from build123d import *

# Parameters (mm, degrees)
EXTRUDE_1_DEPTH             = 3
SKETCH_2_R                  = 1.5
CUT_EXTRUDE_1_DEPTH         = 158.429349233
FILLET_1_R                  = 10
FILLET_2_R                  = 2
HOLE_WIZARD_M3_1_AT_2_COUNT = 2
HOLE_WIZARD_M3_1_AT_2_PITCH = 20


with BuildPart() as part:
    # 草图1 → 凸台-拉伸1 (new body)
    with BuildSketch(Plane.XY):
        Polygon((0, 0), (130, 0), (65, 88.741196746), align=None)
    extrude(amount=EXTRUDE_1_DEPTH)

    # 草图2 → 切除-拉伸1 (cut, through all)
    with BuildSketch(Plane.XY.offset(3)):
        with Locations((42.987595979, 36.688780191)):
            Circle(SKETCH_2_R)
        with Locations(Location((31.169414161, 20.554017147, 0), (0, 0, 180))):
            Circle(SKETCH_2_R)
    extrude(amount=-CUT_EXTRUDE_1_DEPTH, mode=Mode.SUBTRACT)

    # 圆角1
    fillet_1_edges = [part.edges().sort_by_distance(p)[0] for p in [
        (0, 0, 1.5),
    ]]
    fillet(fillet_1_edges, radius=FILLET_1_R)

    # 圆角2
    fillet_2_edges = [part.edges().sort_by_distance(p)[0] for p in [
        (65, 88.741196746, 1.5),
        (130, 0, 1.5),
    ]]
    fillet(fillet_2_edges, radius=FILLET_2_R)

    # 草图6 → M3 六角凹锥坑螺钉的锥形沉头孔1 (revolve, cut)
    with BuildSketch(Plane(origin=(42.987595979, 36.688780191, 3), x_dir=(0, -1, 0), z_dir=(1, 0, 0))):
        Polygon((0, 0), (0, 3), (1.7, 3), (1.7, 1.66), (3.36, 0), align=None)
    hole_wizard_m3_1 = revolve(axis=Axis((42.987595979, 36.688780191, 9.35), (0, 0, -1)), mode=Mode.SUBTRACT)

    # M3 六角凹锥坑螺钉的锥形沉头孔1 at 2: M3 六角凹锥坑螺钉的锥形沉头孔1 ×2
    with Locations(*[Vector(-0.5909090909090912, -0.8067381522408567, 0) * (i * HOLE_WIZARD_M3_1_AT_2_PITCH) for i in range(1, HOLE_WIZARD_M3_1_AT_2_COUNT)]):
        add(hole_wizard_m3_1, mode=Mode.SUBTRACT)


solid = part.part
Geometry: final body of the model. Coordinates: model frame, mm. Give positions to 0.01 mm unless a question says otherwise; leave off trailing zeros. Write each loop counter-clockwise with the first axis right and the second up, starting at its lowest first coordinate (ties: lowest second). Pieces come first, ordered by that corner, then holes.
(1) Cut plane A-A, the plane z = 2.5. Return loops of the section in (x, y), then the cut area to 3 significant figures.
(2) Cut plane C-C, the plane x = 118. Return loops of the section in (y, z), then the cut area to 3 significant figures.
(3) First-contact query: P1, Ø1.5, axis at y = 39.5, z = 1, coming from the +X side. Flat tip, straight axial feed; report the tip coordinate or a pass-through.
(4) Cut plane B-B, the plane y = 46.5. Return loops of the section in (x, z).
(5) Ray query, line 1 (Y direction, x = 93.5, z = 1.05); line 2 (X direction, y = 76.5, z = 0.65); line 3 (Y direction, x = 55, z = 2.5). Return the intervals inside material, ascending.
(6) Mould query, pull axis X, two halves, no side actions, for faces 1 (the cylindrical face through (42.913, 38.387, 0.679)), 2 (the flat face through (97.569, 44.277, 1.479)), 3 (the cylindrical face through (32.68, 19.77, 0.68)), 4 (the cylindrical face through (65.026, 87.356, 1.521)). Classes: released by +X, released by -X, zero draft, split by the parting line, or undercut.
Values follow:
1. outline: (11.65, 15.91) arc R10 ccw to (19.72, 0) - (126.06, 0) arc R2 ccw to (127.67, 3.18) - (66.61, 86.54) arc R2 ccw to (63.39, 86.54) - close; hole circle Ø5.72 at (31.17, 20.55); hole circle Ø5.72 at (42.99, 36.69)
1. area: 5,620 mm2
2. outline: (0, 0) - (16.38, 0) - (16.38, 3) - (0, 3) - close
2. area: 49.1 mm2
3. P1: stops at x = 101.62
4. outline: (34.06, 0) - (95.94, 0) - (95.94, 3) - (34.06, 3) - close
5. line 1: y = 0 to 49.83
5. line 2: x = 56.03 to 73.97
5. line 3: y = 0 to 75.09
6. face 1: undercut
6. face 2: released by +X
6. face 3: undercut
6. face 4: split by the parting line
